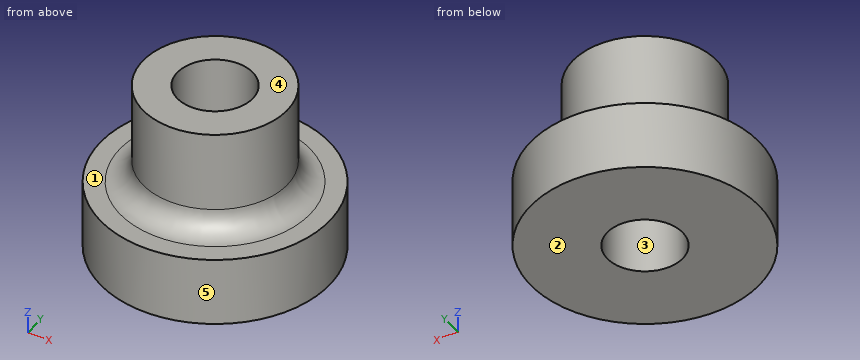
```python
from build123d import *

# Parameters (mm, degrees)
SKETCH1_R           = 3.15
BOSS_EXTRUDE1_DEPTH = 4.5
SKETCH2_R           = 5
BOSS_EXTRUDE2_DEPTH = 3
FILLET1_R           = 1
CUT_EXTRUDE1_REACH  = 12.308
SKETCH3_R           = 1.65


with BuildPart() as part:
    # Sketch1 → Boss-Extrude1 (new body)
    with BuildSketch(Plane.XY):
        Circle(SKETCH1_R)
    extrude(amount=BOSS_EXTRUDE1_DEPTH)

    # Sketch2 → Boss-Extrude2 (add)
    with BuildSketch(Plane(origin=(0, 0, 0), x_dir=(-1, 0, 0), z_dir=(0, 0, -1))):
        Circle(SKETCH2_R)
    extrude(amount=BOSS_EXTRUDE2_DEPTH)

    # Fillet1
    fillet1_edges = [part.edges().sort_by_distance(p)[0] for p in [
        (-3.15, 0, 0),
    ]]
    fillet(fillet1_edges, radius=FILLET1_R)

    # Sketch3 → Cut-Extrude1 (cut, up to next)
    with BuildSketch(Plane(origin=(0, 0, -3), x_dir=(-1, 0, 0), z_dir=(0, 0, -1)), mode=Mode.PRIVATE) as cut_extrude1_sk1:
        Circle(SKETCH3_R)
    cut_extrude1_tool1 = extrude(cut_extrude1_sk1.sketch, amount=-CUT_EXTRUDE1_REACH, mode=Mode.PRIVATE) & part.part
    add(cut_extrude1_tool1.solids().sort_by_distance((0, 0, -3))[0], mode=Mode.SUBTRACT)


solid = part.part
```
Can you work these out from the model? Positions are in its coordinate system, mm. Face numbers are marked on the shaded views. A direction names the side the tool comes from. Round coordinates to 2 decimals unless told otherwise and drop trailing zeros. Loops run counter-clockwise (first coordinate to the right, second up) from the corner with the lowest first, then second, coordinate; pieces in that order, holes last.
Item 1: Will this pin go through, and if not, where does the flat tip stop? pin 1 Ø3 at (y, z) = (3.5, 2) entering from +X.
Item 2: Suppose I cut it at D-D, the plane z = 3. Write out the boundary of the cut face in (x, y).
Item 3: Suppose I cut it at C-C, the plane z = -1.75. Write out the boundary of the cut face in (x, y), then the cut area to 3 significant figures.
Item 4: Please list where these lines run through material, in increasing order: L1, parallel to Y at x = 0, z = 1.25; L2, parallel to Y at x = 0, z = -0.25; L3, parallel to Z at x = -1.5, y = 4.25.
Item 5: Suppose I cut it at A-A, the plane x = 0. Write out the boundary of the cut face in (y, z).
Item 6: If we mould it in two halves opening along Y, with no side actions, what happens to the marked faces 3, 4 and 5? For each: +Y half, -Y half, draft (parallel to the pull), parting line (faces both ways), or undercut.
Item 7: Which directions (+Z, -Z, +X, -X, +Y, -Y) give clear straight access to the entire face, cutting with the end or side of a thin tool? Please do the marked faces 1 and 2.
Reported:
1. pin 1: stops at x = 2.43
2. outline: circle Ø6.3 at (0, 0); hole circle Ø3.3 at (0, 0)
3. outline: circle Ø10 at (0, 0); hole circle Ø3.3 at (0, 0)
3. area: 70.0 mm2
4. L1: y = -3.15 to -1.65, 1.65 to 3.15
4. L2: y = -5 to -1.65, 1.65 to 5
4. L3: z = -3 to 0
5. outline: (-5, -3) - (-1.65, -3) - (-1.65, 4.5) - (-3.15, 4.5) - (-3.15, 1) arc R1 cw to (-4.15, 0) - (-5, 0) - close; (1.65, -3) - (5, -3) - (5, 0) - (4.15, 0) arc R1 cw to (3.15, 1) - (3.15, 4.5) - (1.65, 4.5) - close
6. face 3: undercut
6. face 4: draft
6. face 5: parting line
7. face 1: +Z
7. face 2: -Z, +X, -X, +Y, -Y
